Answer from the drawing. Dimensions are ordinates in mm from the lowest x, y and z of the part. Round coordinates to 2 decimals unless told otherwise and drop trailing zeros. Write each loop counter-clockwise with the first axis right and the second up, starting at its lowest first coordinate (ties: lowest second). Pieces come first, ordered by that corner, then holes. Notation, with made-up numbers: (-25, 76.25) - (24, 76.25) arc R23 ccw to (24, 115.25) - close; hole circle Ø1 at (33.5, -2.5). An arc over 180 degrees is marked (long way). One line per item, written item: value. Start each with the question number.
(1) Find the intervals of material crossed by L1, parallel to X at y = 115, z = 1; L2, parallel to Y at x = 308.5, z = 5.75; L3, parallel to X at y = 68.5, z = 2, in increasing order.
(2) A cutting plane is placed at B-B, the plane y = 130. Determine the outline of the cut face in (x, z), plus the area to 3 significant figures.
(3) A cutting plane is placed at C-C, the plane z = 3.25. Determine the outline of the cut face in (x, y).
(4) A cutting plane is placed at A-A, the plane x = 344.5. Determine the outline of the cut face in (y, z).
(5) A cutting plane is placed at D-D, the plane y = 39.5. Determine the outline of the cut face in (x, z).
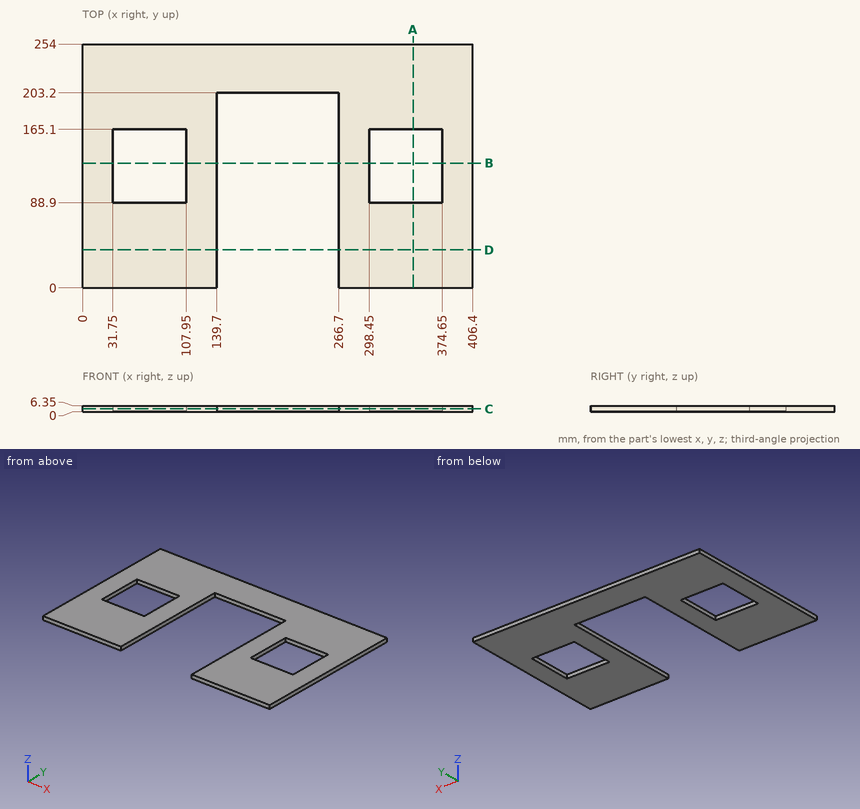
Here are the results:
1. L1: 0 to 31.75, 107.95 to 139.7, 266.7 to 298.45, 374.65 to 406.4
1. L2: 0 to 88.9, 165.1 to 254
1. L3: 0 to 139.7, 266.7 to 406.4
2. outline: (0, 0) - (31.75, 0) - (31.75, 6.35) - (0, 6.35) - close; (107.95, 0) - (139.7, 0) - (139.7, 6.35) - (107.95, 6.35) - close; (266.7, 0) - (298.45, 0) - (298.45, 6.35) - (266.7, 6.35) - close; (374.65, 0) - (406.4, 0) - (406.4, 6.35) - (374.65, 6.35) - close
2. area: 806 mm²
3. outline: (0, 0) - (139.7, 0) - (139.7, 203.2) - (266.7, 203.2) - (266.7, 0) - (406.4, 0) - (406.4, 254) - (0, 254) - close; hole (31.75, 88.9) - (107.95, 88.9) - (107.95, 165.1) - (31.75, 165.1) - close; hole (298.45, 88.9) - (374.65, 88.9) - (374.65, 165.1) - (298.45, 165.1) - close
4. outline: (0, 0) - (88.9, 0) - (88.9, 6.35) - (0, 6.35) - close; (165.1, 0) - (254, 0) - (254, 6.35) - (165.1, 6.35) - close
5. outline: (0, 0) - (139.7, 0) - (139.7, 6.35) - (0, 6.35) - close; (266.7, 0) - (406.4, 0) - (406.4, 6.35) - (266.7, 6.35) - close
